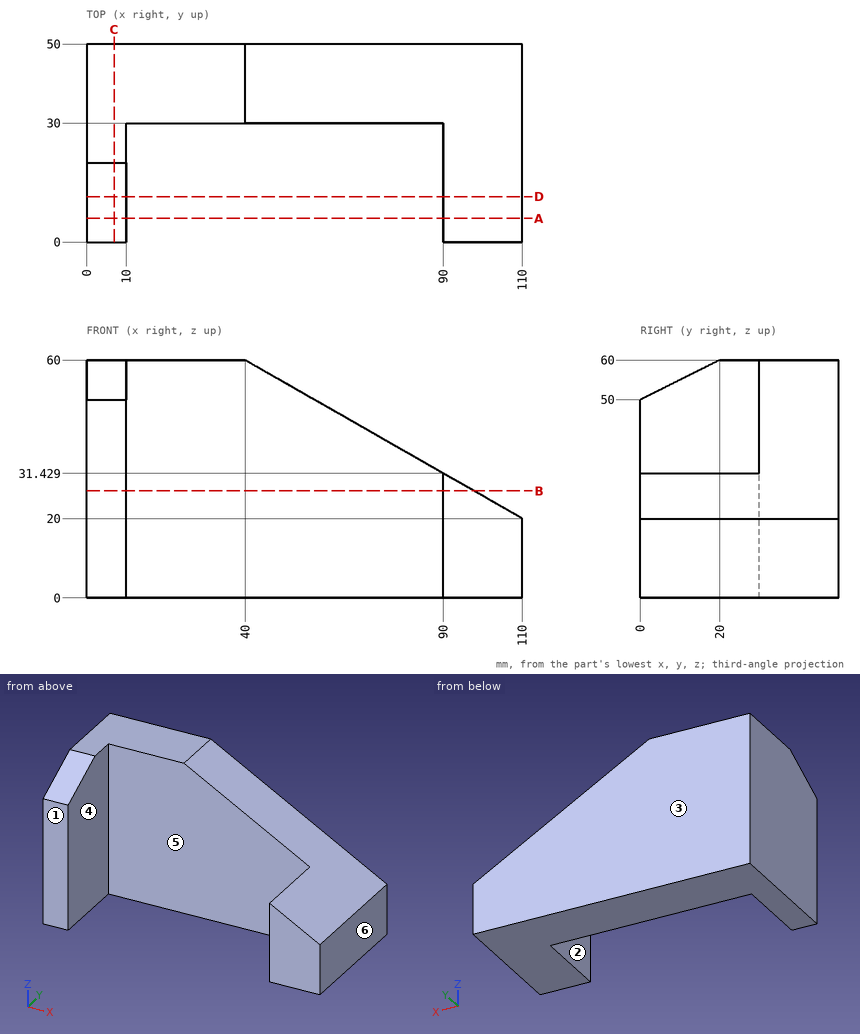
Geometry: see drawing. Coordinates: mm, zero at the bounding-box minimum. A direction names the side the tool comes from. Give positions to 0.01 mm unless a question says otherwise; leave off trailing zeros. Write each loop counter-clockwise with the first axis right and the second up, starting at its lowest first coordinate (ties: lowest second). Pieces come first, ordered by that corner, then holes. Notation, with made-up numbers: M 78,13.25 L 87,13.25 A20 ccw 87,24.25 Z; hole C 10.25,65.25 d5. An arc over 180 degrees is marked long. Answer in a Markdown table with one row per item. Add a question column.
(1) Section A-A on y = 6. Return loops of the section in (x, z).
(2) Section B-B on z = 27. Return loops of the section in (x, y), and give its area (3 significant figures).
(3) Mould query, pull axis X, two halves, no side actions, for the marked faces 3, 4, 5 and 6. Classes: +X half, -X half, draft (parallel to the pull), parting line (faces both ways), or undercut.
(4) Section D-D on y = 11.5. Return loops of the section in (x, z).
(5) Section C-C on x = 7. Return loops of the section in (y, z), and give its area (3 significant figures).
(6) Ray query, line 1 (X direction, y = 28, z = 10); line 2 (Y direction, x = 13.5, z = 32.5); line 3 (X direction, y = 20, z = 28.5) (1 decimal). Return the intervals inside material, ascending.
(7) First-contact query: pin 1 (1 mm diameter, centred on y = 37.5, z = 45.5, fed in from +X); pin 2 (6 mm diameter, centred on x = 82, y = 36, fed in from +Z) (1 decimal); pin 3 (10 mm diameter, centred on y = 6.5, z = 36, fed in from +X); pin 4 (8 mm diameter, centred on x = 84, y = 25, fed in from -Z). Flat tips, straight axial feed; report the tip coordinate or a pass-through.
(8) Reachability of the marked faces 1 and 2 from +Z, -Z, +X, -X, +Y, -Y: full face, straight path, thin tool, end or side. Return the list, or none.
Result set:
| question | item | result |
|---|---|---|
| 1 | outline | M 0,0 L 10,0 L 10,53 L 0,53 Z; M 90,0 L 110,0 L 110,20 L 90,31.43 Z |
| 2 | outline | M 0,0 L 10,0 L 10,30 L 90,30 L 90,0 L 97.75,0 L 97.75,50 L 0,50 Z |
| 2 | area | 2,490 mm^2 |
| 3 | face 3 | draft |
| 3 | face 4 | undercut |
| 3 | face 5 | undercut |
| 3 | face 6 | +X half |
| 4 | outline | M 0,0 L 10,0 L 10,55.75 L 0,55.75 Z; M 90,0 L 110,0 L 110,20 L 90,31.43 Z |
| 5 | outline | M 0,0 L 50,0 L 50,60 L 20,60 L 0,50 Z |
| 5 | area | 2,900 mm^2 |
| 6 | line 1 | x = 0 to 10, 90 to 110 |
| 6 | line 2 | y = 30 to 50 |
| 6 | line 3 | x = 0 to 10, 90 to 95.1 |
| 7 | pin 1 | stops at x = 66.25 |
| 7 | pin 2 | stops at z = 37.7 |
| 7 | pin 3 | stops at x = 90.75 |
| 7 | pin 4 | passes through |
| 8 | face 1 | +Z, -Z, +X, -X, -Y |
| 8 | face 2 | +Z, -Z, -Y |
